Verification items for the finished model (mm, model axes). A direction names the side the tool comes from. Give positions to 0.01 mm unless a question says otherwise; leave off trailing zeros. Loops run counter-clockwise (first coordinate to the right, second up) from the corner with the lowest first, then second, coordinate; pieces in that order, holes last. Notation, with made-up numbers: M -21.75,18.25 L -4.75,18.25 A36 cw -4.75,55.25 Z; hole C 22.25,17 d5. An arc over 180 degrees is marked long. Put each result on its own line as item: value. Start each with the question number.
from build123d import *

# Parameters (mm, degrees)
UPPER_PERIMETER_START                         = 304
SKETCH1_W                                     = 220
SKETCH1_H                                     = 180
SKETCH1_W_2                                   = 200
SKETCH1_H_2                                   = 160
UPPER_PERIMETER_DEPTH                         = 4
BEARING_SPINE_START                           = 304
SKETCH2_W                                     = 10
SKETCH2_H                                     = 170
BEARING_SPINE_DEPTH                           = 4
UPPER_OUTER_RACE_STOP_START                   = 299.9
SKETCH3_R                                     = 11
SKETCH3_R_2                                   = 5.7
UPPER_OUTER_RACE_STOP_DEPTH                   = 8.1
FLOATING_OUTER_RACE_SEAT_START                = 294.5
SKETCH4_R                                     = 10
SKETCH4_R_2                                   = 6.5
FLOATING_OUTER_RACE_SEAT_DEPTH                = 5.41
SHAFT_CLIP_CLEARANCE_START                    = -8.11
SKETCH5_R                                     = 5.7
SHAFT_CLIP_CLEARANCE_DEPTH                    = 8.11
SKETCH6_R                                     = 1.7
FOUR_TIE_ROD_CLEARANCE_DEPTH                  = 4.01
SKETCH7_R                                     = 1
THREE_M2_TOP_CAP_THREAD_MAJOR_ENVELOPES_DEPTH = 4.3
SKETCH8_R                                     = 1.7
BENCH_MOTOR_CROSSBEAM_FOUR_D3P4_DEPTH         = 4.01


with BuildPart() as part:
    # Sketch1 → Upper_Perimeter (new body)
    with BuildSketch(Plane.XY.offset(UPPER_PERIMETER_START)):
        Rectangle(SKETCH1_W, SKETCH1_H)
        Rectangle(SKETCH1_W_2, SKETCH1_H_2, mode=Mode.SUBTRACT)
    extrude(amount=UPPER_PERIMETER_DEPTH)

    # Sketch2 → Bearing_Spine (add)
    with BuildSketch(Plane.XY.offset(BEARING_SPINE_START)):
        Rectangle(SKETCH2_W, SKETCH2_H)
    extrude(amount=BEARING_SPINE_DEPTH)

    # Sketch3 → Upper_Outer_Race_Stop (add)
    with BuildSketch(Plane.XY.offset(UPPER_OUTER_RACE_STOP_START)):
        with Locations(Location((0, 0, 0), (0, 0, 117.035691789))):
            Circle(SKETCH3_R)
        with Locations(Location((0, 0, 0), (0, 0, 208.694413527))):
            Circle(SKETCH3_R_2, mode=Mode.SUBTRACT)
    extrude(amount=UPPER_OUTER_RACE_STOP_DEPTH)

    # Sketch4 → Floating_Outer_Race_Seat (add)
    with BuildSketch(Plane.XY.offset(FLOATING_OUTER_RACE_SEAT_START)):
        Circle(SKETCH4_R)
        Circle(SKETCH4_R_2, mode=Mode.SUBTRACT)
    extrude(amount=FLOATING_OUTER_RACE_SEAT_DEPTH)

    # Sketch5 → Shaft_Clip_Clearance (cut)
    with BuildSketch(Plane.XY.offset(308).offset(SHAFT_CLIP_CLEARANCE_START)):
        Circle(SKETCH5_R)
    extrude(amount=SHAFT_CLIP_CLEARANCE_DEPTH, mode=Mode.SUBTRACT)

    # Sketch6 → Four_Tie_Rod_Clearance (cut)
    with BuildSketch(Plane.XY.offset(308)):
        with Locations((-105, -85)):
            Circle(SKETCH6_R)
        with Locations((-105, 85)):
            Circle(SKETCH6_R)
        with Locations((105, -85)):
            Circle(SKETCH6_R)
        with Locations((105, 85)):
            Circle(SKETCH6_R)
    extrude(amount=-FOUR_TIE_ROD_CLEARANCE_DEPTH, mode=Mode.SUBTRACT)

    # Sketch7 → Three_M2_Top_Cap_Thread_Major_Envelopes (cut)
    with BuildSketch(Plane(origin=(0, 0, 294.5), x_dir=(-1, 0, 0), z_dir=(0, 0, -1))):
        with Locations((-7.188010851, 4.15)):
            Circle(SKETCH7_R)
        with Locations((7.188010851, 4.15)):
            Circle(SKETCH7_R)
        with Locations((0, -8.3)):
            Circle(SKETCH7_R)
    extrude(amount=-THREE_M2_TOP_CAP_THREAD_MAJOR_ENVELOPES_DEPTH, mode=Mode.SUBTRACT)

    # Sketch8 → Bench_Motor_Crossbeam_Four_D3p4 (cut)
    with BuildSketch(Plane.XY.offset(308)):
        with Locations((-105, -36)):
            Circle(SKETCH8_R)
        with Locations((-105, 36)):
            Circle(SKETCH8_R)
        with Locations((105, -36)):
            Circle(SKETCH8_R)
        with Locations((105, 36)):
            Circle(SKETCH8_R)
    extrude(amount=-BENCH_MOTOR_CROSSBEAM_FOUR_D3P4_DEPTH, mode=Mode.SUBTRACT)


solid = part.part
Q1. Set-up check for faces 1 (the face through (-5.158, -3.955, 297.162)), 2 (the face through (0, -7, 294.5)): record each of +Z, -Z, +X, -X, +Y, -Y from which the full face is reachable in a straight line by a thin tool's end or side.
Q2. Release check for a two-part mould opening along Y. For faces 3 (the face through (8, 7, 299.9)), 4 (the face through (-2.17, -9.76, 297.16)), 5 (the face through (-0.866, 10.966, 302.993)) record: pulls with the +Y half, pulls with the -Y half, needs draft (parallel to the pull), parting line crosses it, or undercut.
Q3. Scan lines: L1, parallel to X at y = -23, z = 306; L2, parallel to Y at x = -105, z = 305.9; L3, parallel to Y at x = 0, z = 296.35. Record each from-to range of solid material in increasing order.
Q4. Go/stop test with flat-tipped pins: pin 1 (5 mm diameter, centred on y = -44.5, z = 300.5, fed in from +X); pin 2 (3 mm diameter, centred on x = 2.5, z = 296.5, fed in from +Y); pin 3 (1.6 mm diameter, centred on x = 7.19, y = 4.15, fed in from -Z). Record where each tip stops, or that it passes through.
Q5. Cross-section at B-B, the plane y = -24. Record the boundary of the cut face in (x, z).
Q6. Cross-section at A-A, the plane x = 59. Record the boundary of the cut face in (y, z), then the cut area to 3 significant figures.
Ans:
1. face 1: -Z
1. face 2: -Z, +X, -X, +Y, -Y
2. face 3: needs draft
2. face 4: parting line crosses it
2. face 5: undercut
3. L1: x = -110 to -100, -5 to 5, 100 to 110
3. L2: y = -90 to -86.7, -83.3 to -37.7, -34.3 to 34.3, 37.7 to 83.3, 86.7 to 90
3. L3: y = -10 to -9.3, -7.3 to -6.5, 6.5 to 10
4. pin 1: passes through
4. pin 2: stops at y = 9.95
4. pin 3: stops at z = 298.8
5. outline: M -110,304 L -100,304 L -100,308 L -110,308 Z; M -5,304 L 5,304 L 5,308 L -5,308 Z; M 100,304 L 110,304 L 110,308 L 100,308 Z
6. outline: M -90,304 L -80,304 L -80,308 L -90,308 Z; M 80,304 L 90,304 L 90,308 L 80,308 Z
6. area: 80.0 mm^2
